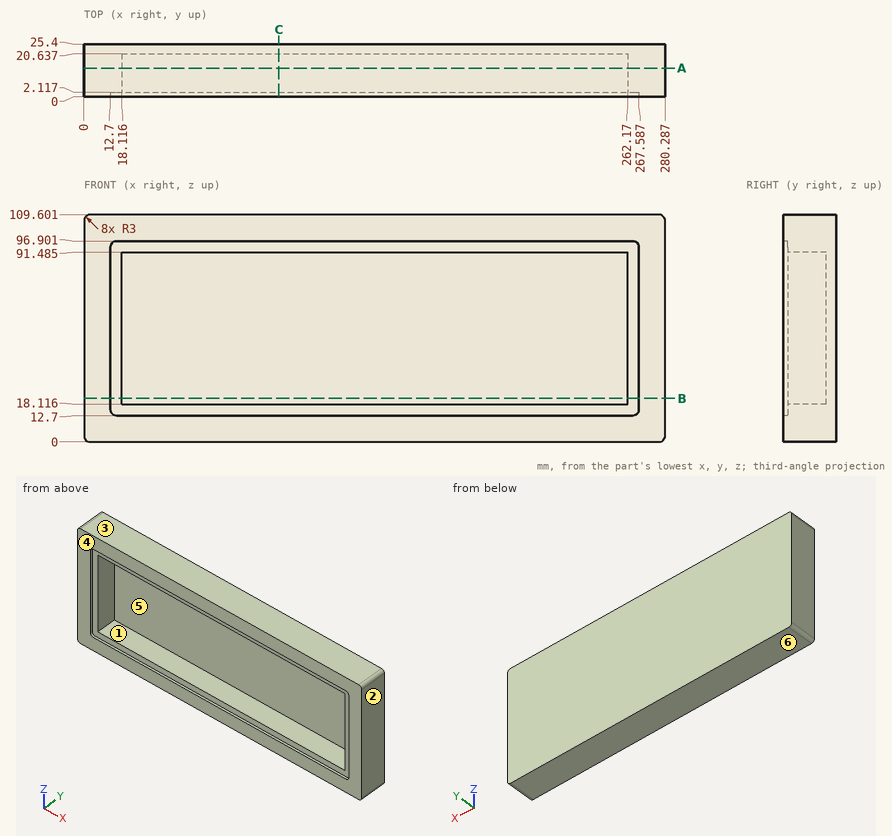
Job drawing, mm, ordinate dimensions from the low corner. One solid piece. A direction names the side the tool comes from. Coordinates: 2 decimals unless noted, no trailing zeros. Order: outer loops, then holes, each group sorted by start corner. A loop starts at its lowest first (then second) coordinate and runs counter-clockwise, first axis right, second up. Notation, with made-up numbers: (55, 6) - (80, 6) arc R28 cw to (80, 29) - close; hole circle Ø2 at (30, 24.25). An arc over 180 degrees is marked (long way). Use CSV: the item, a comma, the result in double quotes.
Item 1: Saw through at A-A on y = 13.75. Give the cut face in (x, z) (1 decimal).
Solved:
outline,"(0, 3) arc R3 ccw to (3, 0) - (277.3, 0) arc R3 ccw to (280.3, 3) - (280.3, 106.6) arc R3 ccw to (277.3, 109.6) - (3, 109.6) arc R3 ccw to (0, 106.6) - close; hole (18.1, 18.1) - (262.2, 18.1) - (262.2, 91.5) - (18.1, 91.5) - close"
Item 2: Drop a flat-ended pin along its axis: P1, Ø3, axis at x = 122, z = 56.5, coming from the -Y side. Give the stop position or say it passes through.
Solved:
P1,"stops at y = 20.64"
Item 3: 3-axis set-ups, long thin cutter, end or side, ignore diameter. For the marked faces 1 and 2: which of +Z, -Z, +X, -X, +Y, -Y reach the whole face in a straight line?
Solved:
face 1,"-Y"
face 2,"+Z, -Z, +X, +Y, -Y"
Item 4: Probe probe 1 along X at (y, z) = (10, 60); probe 2 along Z at (x, y) = (176.5, 8.25) (1 decimal); probe 3 along X at (y, z) = (1.25, 70.5). List the from-to ranges inside material, lowest first.
Solved:
probe 1,"x = 0 to 18.12, 262.17 to 280.29"
probe 2,"z = 0 to 18.1, 91.5 to 109.6"
probe 3,"x = 0 to 12.7, 267.59 to 280.29"
Item 5: Saw through at B-B on z = 21. Give the cut face in (x, y), and give its area (3 significant figures).
Solved:
outline,"(0, 0) - (12.7, 0) - (12.7, 2.12) - (18.12, 2.12) - (18.12, 20.64) - (262.17, 20.64) - (262.17, 2.12) - (267.59, 2.12) - (267.59, 0) - (280.29, 0) - (280.29, 25.4) - (0, 25.4) - close"
area,"2,060 mm²"
Item 6: Mould opens along Z. For the marked faces 3, 4, 5 and 6 say: +Z half, -Z half, draft (parallel to the pull), parting line (faces both ways), or undercut.
Solved:
face 3,"+Z half"
face 4,"draft"
face 5,"undercut"
face 6,"-Z half"
Item 7: Saw through at C-C on x = 94. Give the cut face in (y, z) (1 decimal).
Solved:
outline,"(0, 0) - (25.4, 0) - (25.4, 109.6) - (0, 109.6) - (0, 96.9) - (2.1, 96.9) - (2.1, 91.5) - (20.6, 91.5) - (20.6, 18.1) - (2.1, 18.1) - (2.1, 12.7) - (0, 12.7) - close"
